Could you check a few things on this model? Use its own coordinates, in mm. Face numbers are marked on the shaded views. A direction names the side the tool comes from. Round coordinates to 2 decimals unless told otherwise and drop trailing zeros. Order: outer loops, then holes, each group sorted by start corner. A loop starts at its lowest first (then second) coordinate and runs counter-clockwise, first axis right, second up. Notation, with made-up numbers: (66, -15) - (112, -15) arc R32 cw to (112, 22) - close; hole circle Ø5 at (58.5, -32). An arc over 180 degrees is marked (long way). Use one line per item in the form item = value.
from build123d import *

# Parameters (mm, degrees)
ESQUISSE1_W      = 104
ESQUISSE1_H      = 81
ESQUISSE1_R      = 1.55
EXTRUSION2_DEPTH = 1.55
ESQUISSE2_W      = 51.46
ESQUISSE2_H      = 4.95
EXTRUSION3_DEPTH = 12.6
ESQUISSE3_W      = 5.8
ESQUISSE3_H      = 10.16
EXTRUSION4_DEPTH = 11.7
ESQUISSE4_W      = 5.8
ESQUISSE4_H      = 10.16
EXTRUSION5_DEPTH = 11.7


with BuildPart() as part:
    # Esquisse1 → Extrusion2 (new body)
    with BuildSketch(Plane(origin=(0, 0, 0), x_dir=(1, 0, 0), z_dir=(0, 1, 0))):
        with Locations((31, 37)):
            Rectangle(ESQUISSE1_W, ESQUISSE1_H)
        with Locations((-17, 1.27)):
            Circle(ESQUISSE1_R, mode=Mode.SUBTRACT)
        with Locations((-17, 72)):
            Circle(ESQUISSE1_R, mode=Mode.SUBTRACT)
        with Locations((74, 72)):
            Circle(ESQUISSE1_R, mode=Mode.SUBTRACT)
        with Locations((74, 1.27)):
            Circle(ESQUISSE1_R, mode=Mode.SUBTRACT)
    extrude(amount=EXTRUSION2_DEPTH)

    # Esquisse2 → Extrusion3 (add)
    with BuildSketch(Plane(origin=(0, 1.55, 0), x_dir=(-1, 0, 0), z_dir=(0, 1, 0))):
        with Locations((-24.13, -72)):
            Rectangle(ESQUISSE2_W, ESQUISSE2_H)
        with Locations((-24.13, -1.27)):
            Rectangle(ESQUISSE2_W, ESQUISSE2_H)
    extrude(amount=-EXTRUSION3_DEPTH)

    # Esquisse3 → Extrusion4 (add)
    with BuildSketch(Plane(origin=(0, 1.55, 0), x_dir=(-1, 0, 0), z_dir=(0, 1, 0))):
        with Locations((10, -31.23)):
            Rectangle(ESQUISSE3_W, ESQUISSE3_H)
        with Locations((10, -14.23)):
            Rectangle(ESQUISSE3_W, ESQUISSE3_H)
        with Locations((10, -46.282)):
            Rectangle(ESQUISSE3_W, ESQUISSE3_H)
    extrude(amount=EXTRUSION4_DEPTH)

    # Esquisse4 → Extrusion5 (add)
    with BuildSketch(Plane(origin=(0, 1.55, 0), x_dir=(-1, 0, 0), z_dir=(0, 1, 0))):
        with Locations((-69.9, -10.91)):
            Rectangle(ESQUISSE4_W, ESQUISSE4_H)
        with Locations((-76, -10.91)):
            Rectangle(ESQUISSE4_W, ESQUISSE4_H)
        with Locations((-69.825093766, -25.51)):
            Rectangle(ESQUISSE4_W, ESQUISSE4_H)
        with Locations((-75.925093766, -25.51)):
            Rectangle(ESQUISSE4_W, ESQUISSE4_H)
    extrude(amount=EXTRUSION5_DEPTH)


solid = part.part
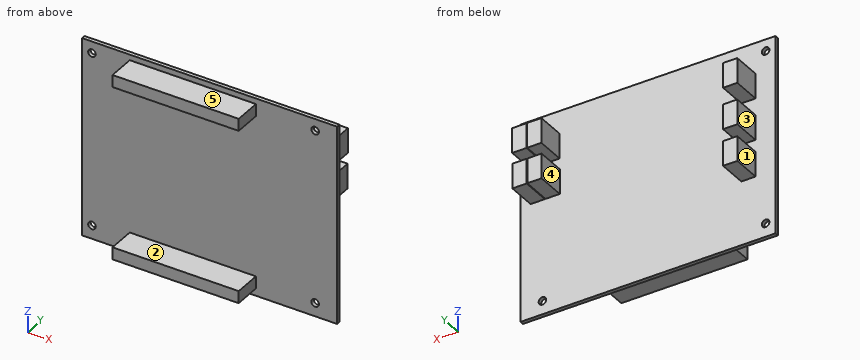
Item 1: If we mould it in two halves opening along X, with no side actions, what happens to the marked faces 3, 4 and 5? For each: released by +X, released by -X, zero draft, split by the parting line, or undercut.
Found:
face_3 = released by -X
face_4 = undercut
face_5 = zero draft
Item 2: I need wall thicknesses on L1, parallel to Z at x = -17, y = 0.35; L2, parallel to X at y = 0.4, z = -72; L3, parallel to Z at x = 78.5, y = 8.5. Which ranges of each line are inside material? Lowest first, please.
Found:
L1 = -77.5 to -73.55, -70.45 to -2.82, 0.28 to 3.5
L2 = -21 to -18.55, -15.45 to 72.45, 75.55 to 83
L3 = -30.59 to -20.43, -15.99 to -5.83
Item 3: Will these pins go through, and if not, where does the flat tip stop? P1, Ø1.7, axis at x = -9.5, y = 9, coming from the +Z side; P2, Ø3, axis at x = -11, y = 9, coming from the -Z side; P3, Ø12, axis at x = 18.5, y = -4.5, coming from the +Z side; P4, Ø1.5, axis at x = 64, z = -68, coming from the +Y side.
Found:
P1 = -9.15
P2 = -51.36
P3 = 3.5
P4 = 1.55
Item 4: For the marked faces 1 and 2, which set-ups out of +Z, -Z, +X, -X, +Y, -Y let a thin tool reach every point of the face, with its end or its side?
Found:
face_1 = +Z, -Z, -X, +Y
face_2 = +X, -X, -Y
Item 5: Imagine slicing it at B-B on z = -1.27. Please give me the cut outline in (x, y), plus the area to 3 significant figures.
Found:
outline = (-21, 0) - (-18.55, 0) - (-18.55, 1.55) - (-21, 1.55) - close; (-15.45, 0) - (-1.6, 0) - (-1.6, -11.05) - (49.86, -11.05) - (49.86, 0) - (72.45, 0) - (72.45, 1.55) - (-15.45, 1.55) - close; (75.55, 0) - (83, 0) - (83, 1.55) - (75.55, 1.55) - close
area = 720 mm2
Item 6: Imagine slicing it at D-D on z = -47. Please give me the cut outline in (x, y).
Found:
outline = (-21, 0) - (83, 0) - (83, 1.55) - (-7.1, 1.55) - (-7.1, 13.25) - (-12.9, 13.25) - (-12.9, 1.55) - (-21, 1.55) - close
Item 7: Imagine slicing it at C-C on y = -5.25. Please give me the cut outline in (x, z) (3 decimals), plus the area to 3 significant figures.
Found:
outline = (-1.6, -74.475) - (49.86, -74.475) - (49.86, -69.525) - (-1.6, -69.525) - close; (-1.6, -3.745) - (49.86, -3.745) - (49.86, 1.205) - (-1.6, 1.205) - close
area = 509 mm2
Item 8: Imagine slicing it at A-A on y = 11.75. Please give me the cut outline in (x, z), plus the area to 3 significant figures.
Found:
outline = (-12.9, -51.36) - (-7.1, -51.36) - (-7.1, -41.2) - (-12.9, -41.2) - close; (-12.9, -36.31) - (-7.1, -36.31) - (-7.1, -26.15) - (-12.9, -26.15) - close; (-12.9, -19.31) - (-7.1, -19.31) - (-7.1, -9.15) - (-12.9, -9.15) - close; (66.93, -30.59) - (72.73, -30.59) - (72.73, -20.43) - (66.93, -20.43) - close; (67, -15.99) - (72.8, -15.99) - (72.8, -5.83) - (67, -5.83) - close; (73.03, -30.59) - (78.83, -30.59) - (78.83, -20.43) - (73.03, -20.43) - close; (73.1, -15.99) - (78.9, -15.99) - (78.9, -5.83) - (73.1, -5.83) - close
area = 412 mm2
